Could you check a few things on this model? Use its own coordinates, in mm. A direction names the side the tool comes from. Coordinates: 2 decimals unless noted, no trailing zeros. Order: outer loops, then holes, each group sorted by start corner. A loop starts at its lowest first (then second) coordinate and runs counter-clockwise, first axis right, second up. Notation, with made-up numbers: (4.25, 15.25) - (45.25, 15.25) arc R30 cw to (45.25, 50.25) - close; hole circle Ø9 at (12, -31.5). An arc over 180 degrees is marked (long way). One line per item, written item: value.
from build123d import *

# Parameters (mm, degrees)
SKETCH1_W           = 50
SKETCH1_H           = 42
BOSS_EXTRUDE1_DEPTH = 5
SKETCH2_W           = 5
SKETCH2_H           = 42
BOSS_EXTRUDE2_DEPTH = 45
CUT_EXTRUDE1_DEPTH  = 45
CUT_EXTRUDE3_DEPTH  = 6
SKETCH7_R           = 11
SKETCH7_R_2         = 1.65
SKETCH7_R_3         = 1.5
CUT_EXTRUDE4_DEPTH  = 6


with BuildPart() as part:
    # Sketch1 → Boss-Extrude1 (new body)
    with BuildSketch(Plane(origin=(0, 0, 0), x_dir=(1, 0, 0), z_dir=(0, 1, 0))):
        with Locations((25, 21)):
            Rectangle(SKETCH1_W, SKETCH1_H)
    extrude(amount=BOSS_EXTRUDE1_DEPTH)

    # Sketch2 → Boss-Extrude2 (add)
    with BuildSketch(Plane(origin=(0, 5, 0), x_dir=(1, 0, 0), z_dir=(0, 1, 0))):
        with Locations((2.5, 21)):
            Rectangle(SKETCH2_W, SKETCH2_H)
    extrude(amount=BOSS_EXTRUDE2_DEPTH)

    # Sketch3 → Cut-Extrude1 (cut)
    with BuildSketch(Plane(origin=(5, 0, 0), x_dir=(0, 0, -1), z_dir=(1, 0, 0))):
        Polygon((0, 47), (3, 50), (0, 50), align=None)
        Polygon((42, 50), (39, 50), (42, 47), align=None)
    extrude(amount=-CUT_EXTRUDE1_DEPTH, mode=Mode.SUBTRACT)

    # Sketch4 → Cut-Extrude3 (cut, through all)
    with BuildSketch(Plane(origin=(0, 5, 0), x_dir=(1, 0, 0), z_dir=(0, 1, 0))):
        with BuildLine():
            Line((12.471581484, 8.5), (42.25, 8.5))
            ThreePointArc((42.25, 8.5), (44.5, 6.25), (42.25, 4))
            Line((42.25, 4), (12.471581484, 4))
            ThreePointArc((12.471581484, 4), (9.701111334, 6.25), (12.471581484, 8.5))
        make_face()
        with BuildLine():
            Line((12.471581484, 38), (42.25, 38))
            ThreePointArc((42.25, 38), (44.5, 35.75), (42.25, 33.5))
            Line((42.25, 33.5), (12.471581484, 33.5))
            ThreePointArc((12.471581484, 33.5), (9.701111334, 35.75), (12.471581484, 38))
        make_face()
    extrude(amount=-CUT_EXTRUDE3_DEPTH, mode=Mode.SUBTRACT)

    # Sketch7 → Cut-Extrude4 (cut, through all)
    with BuildSketch(Plane(origin=(5, 0, 0), x_dir=(0, 0, -1), z_dir=(1, 0, 0))):
        with Locations((21, 29.5)):
            Circle(SKETCH7_R)
        with Locations((5.5, 45)):
            Circle(SKETCH7_R_2)
        with Locations((31, 39.5)):
            Circle(SKETCH7_R_3)
        with Locations((5.5, 14)):
            Circle(SKETCH7_R_2)
        with Locations((31, 19.5)):
            Circle(SKETCH7_R_3)
        with Locations((36.5, 14)):
            Circle(SKETCH7_R_2)
        with Locations((11, 19.5)):
            Circle(SKETCH7_R_3)
        with Locations((11, 39.5)):
            Circle(SKETCH7_R_3)
        with Locations((36.5, 45)):
            Circle(SKETCH7_R_2)
    extrude(amount=-CUT_EXTRUDE4_DEPTH, mode=Mode.SUBTRACT)


solid = part.part
Item 1: For faces 4 (the face through (2.54, 14.07, -34.85)), 5 (the face through (5, 17, -21)), 6 (the face through (28, 3, -4)), which set-ups out of +Z, -Z, +X, -X, +Y, -Y let a thin tool reach every point of the face, with its end or its side?
Conclusion:
face 4: +X, -X
face 5: +Z, -Z, +X, +Y
face 6: +Y, -Y
Item 2: I want a section at D-D on x = 3.5. Give the number of separate pieces and of enclosed holes in the cut face, then the cut area to 3 significant figures.
Conclusion:
separate pieces: 1
enclosed holes: 9
area: 1,650 mm²
Item 3: Thinking about a two-plate mould opening in Y: for faces 1 (the face through (2.54, 14.07, -3.85)), 2 (the face through (27, 3, -38)), 3 (the face through (3, 49, -40)), which applies, pulls with the +Y half, pulls with the -Y half, needs draft (parallel to the pull), parting line crosses it, or undercut?
Conclusion:
face 1: undercut
face 2: needs draft
face 3: pulls with the +Y half
Item 4: I want a section at B-B on y = 29.5. Please give me the cut outline in (x, z).
Conclusion:
outline: (0, -42) - (5, -42) - (5, -32) - (0, -32) - close; (0, -10) - (5, -10) - (5, 0) - (0, 0) - close
Item 5: I want a section at A-A on x = 14. Please give me the cut outline in (y, z), then the cut area to 3 significant figures.
Conclusion:
outline: (0, -42) - (5, -42) - (5, -38) - (0, -38) - close; (0, -33.5) - (5, -33.5) - (5, -8.5) - (0, -8.5) - close; (0, -4) - (5, -4) - (5, 0) - (0, 0) - close
area: 165 mm²
Item 6: If I drill on probe 1 along X at (y, z) = (2.5, -6.25); probe 2 along X at (y, z) = (35.5, -35), over which ranges is the centre line in solid material (lowest first)?
Conclusion:
probe 1: 0 to 9.7, 44.5 to 50
probe 2: 0 to 5
Item 7: I'm going to push flat-ended pins straight in: pin 1 Ø6 at (x, z) = (12, -35.75) entering from +Y; pin 2 Ø4 at (y, z) = (39.5, -11) entering from +X; pin 3 Ø2 at (y, z) = (14, -36.5) entering from +X. Where does each tip first touch, or does it pass through?
Conclusion:
pin 1: y = 5
pin 2: x = 5
pin 3: through
Item 8: I want a section at C-C on y = 4. Please give me the cut outline in (x, z), then the cut area to 3 significant figures.
Conclusion:
outline: (0, -42) - (50, -42) - (50, 0) - (0, 0) - close; hole (12.47, -38) - (42.25, -38) arc R2.25 ccw to (42.25, -33.5) - (12.47, -33.5) arc R2.3 ccw (long way) to start; hole (12.47, -8.5) - (42.25, -8.5) arc R2.25 ccw to (42.25, -4) - (12.47, -4) arc R2.3 ccw (long way) to start
area: 1,800 mm²
